Read the model definition and answer for the solid it produces. Units are mm, in the model's axes. Give positions to 0.01 mm unless a question says otherwise; leave off trailing zeros. Order: outer loops, then holes, each group sorted by start corner. A loop starts at its lowest first (then second) coordinate and runs counter-clockwise, first axis right, second up.
Item 1: A cutting plane is placed at C-C (x = -0.5). Write down the section's boundary in (y, z).
Item 2: Find the intervals of material crossed by line 1 along Z through (x, y) = (36, 0.2); line 2 along X through (y, z) = (-0.05, -0.5); line 3 along Z through (x, y) = (-47, -0.7), in increasing order.
Item 3: A cutting plane is placed at B-B (z = 42). Write down the section's boundary in (x, y).
Item 4: A cutting plane is placed at A-A (y = 0). Write down the section's boundary in (x, z), plus the area to 3 significant figures.
from build123d import *

# Parameters (mm, degrees)
SKETCH2_R = 0.9906


with BuildPart() as part:
    # Sweep1: sweep along a path in Sketch1
    with BuildLine(Plane(origin=(0, 0, 0), x_dir=(1, 0, 0), z_dir=(0, 1, 0))) as sweep1_path:
        Line((66.275827552, -58.889759794), (66.275827552, 71.110240206))
        ThreePointArc((66.275827552, 71.110240206), (58.355934841, 90.2305526), (39.235622447, 98.150445311))
        Line((39.235622447, 98.150445311), (-50.764377553, 98.150445311))
        ThreePointArc((-50.764377553, 98.150445311), (-69.884689947, 90.2305526), (-77.804582658, 71.110240206))
        Line((-77.804582658, 71.110240206), (-77.804582658, -58.889759794))
        ThreePointArc((-77.804582658, -58.889759794), (-69.884689947, -78.010072188), (-50.764377553, -85.929964899))
        Line((-50.764377553, -85.929964899), (39.235622447, -85.929964899))
        ThreePointArc((39.235622447, -85.929964899), (58.355934841, -78.010072188), (66.275827552, -58.889759794))
    # Sketch2 → Sweep1 (sweep)
    with BuildSketch(Plane(origin=(66.275827552, 0, -71.110240206), x_dir=(-1, 0, 0), z_dir=(0, 0, -1))):
        Circle(SKETCH2_R)
    sweep(path=sweep1_path.line)


solid = part.part
Response values:
1. outline: circle Ø1.98 at (0, -98.15); circle Ø1.98 at (0, 85.93)
2. line 1: z = -99.12 to -97.18, 84.96 to 86.9
2. line 2: x = -78.79 to -76.82, 65.29 to 67.27
2. line 3: z = -98.85 to -97.45, 85.23 to 86.63
3. outline: circle Ø1.98 at (-77.8, 0); circle Ø1.98 at (66.28, 0)
4. outline: (-78.8, -71.11) arc R28.03 ccw to (-50.76, -99.14) - (39.24, -99.14) arc R28.03 ccw to (67.27, -71.11) - (67.27, 58.89) arc R28.03 ccw to (39.24, 86.92) - (-50.76, 86.92) arc R28.03 ccw to (-78.8, 58.89) - close; hole (-76.81, -71.11) arc R26.05 ccw to (-50.76, -97.16) - (39.24, -97.16) arc R26.05 ccw to (65.29, -71.11) - (65.29, 58.89) arc R26.05 ccw to (39.24, 84.94) - (-50.76, 84.94) arc R26.05 ccw to (-76.81, 58.89) - close
4. area: 1,210 mm2
